```python
from build123d import *

# Parameters (mm, degrees)
SKETCH2_R           = 2.5
BOSS_EXTRUDE1_DEPTH = 2.5
CIRPATTERN1_COUNT   = 3


with BuildPart() as part:
    # Sketch1 → Revolve1 (revolve)
    with BuildSketch(Plane.XY, mode=Mode.PRIVATE) as revolve1_sk:
        Polygon((49.97067965, 0), (52.495498156, 10), (44.195498156, 10), (40, 5), (0, 5), (0, 0), align=None)
    revolve(revolve1_sk.sketch.rotate(Axis((-81.869594145, 0, 0), (1, 0, 0)), 90), axis=Axis((-81.869594145, 0, 0), (1, 0, 0)))



with BuildPart() as body_2:
    # Sketch2 → Revolve2 (revolve)
    with BuildSketch(Plane.XY, mode=Mode.PRIVATE) as revolve2_sk:
        with Locations((55, 31.25)):
            Circle(SKETCH2_R)
    revolve(revolve2_sk.sketch.rotate(Axis((0, 0, 0), (1, 0, 0)), 270), axis=Axis((0, 0, 0), (1, 0, 0)))


with BuildPart() as part_1:
    add(part.part)

    add(body_2.part)  # Boss-Extrude1 merges body 2
    # Sketch3 → Boss-Extrude1 (add, symmetric)
    with BuildSketch(Plane.XY):
        Polygon((51.6, 9.2), (49.554391748, 9.2), (53.974391748, 29.779681075), (56.02, 29.779681075), align=None)
    boss_extrude1 = extrude(amount=BOSS_EXTRUDE1_DEPTH, both=True)

    # CirPattern1: Boss-Extrude1 ×3 about axis
    cirpattern1_axis = Axis((0, 0, 0), (1, 0, 0))
    for i in range(1, CIRPATTERN1_COUNT):
        add(boss_extrude1.rotate(cirpattern1_axis, i * 360 / CIRPATTERN1_COUNT))


solid = part_1.part
```
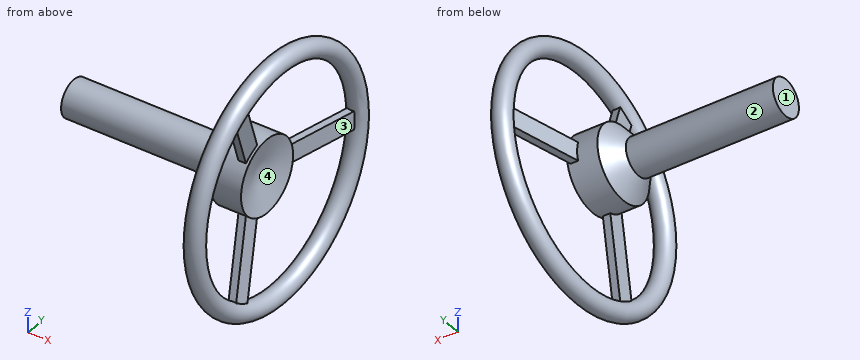
Geometry: final body of the model. Coordinates: model frame, mm. Face numbers are marked on the shaded views. Round coordinates to 2 decimals unless told otherwise and drop trailing zeros. Order: outer loops, then holes, each group sorted by start corner. A loop starts at its lowest first (then second) coordinate and runs counter-clockwise, first axis right, second up. Notation, with made-up numbers: (-37, 44) -> (-10, 44) arc R13 ccw to (-10, 57) -> close; hole circle Ø6 at (42.5, 88). An arc over 180 degrees is marked (long way). Write each question's results on one line, items separated by ' | '.
Q1. Ray query, line 1 along X through (y, z) = (-13.5, 22); line 2 along X through (y, z) = (7, -7); line 3 along Y through (x, z) = (48.5, 3). Return the intervals inside material, ascending.
Response values:
line 1: 53.12 to 55.17 | line 2: 44.11 to 52.47 | line 3: -9.54 to 9.54
Q2. Section query A-A (x = 25.5). Output: boundary loops of the cut face in (y, z).
Response values:
outline: circle Ø10 at (0, 0)
Q3. Pin query (flat end, axial travel): pin 1 Ø3 at (y, z) = (-15.5, 23) entering from +X; pin 2 Ø12 at (y, z) = (-26, 7) entering from +X; pin 3 Ø1.8 at (x, y) = (53, 19.5) entering from +Z; pin 4 Ø7 at (x, y) = (52.5, 21.5) entering from -Z. Return the tip coordinate at first contact, or that it passes through.
Response values:
pin 1: x = 56.48 | pin 2: x = 57.5 | pin 3: z = 27.5 | pin 4: z = -28.11
Q4. Pull-direction query (Y, two-part tool) for the marked faces 1, 2, 3 and 4; classes: released by +Y, released by -Y, zero draft, split by the parting line, or undercut.
Response values:
face 1: zero draft | face 2: split by the parting line | face 3: undercut | face 4: undercut
Q5. Section query D-D (x = 46.5). Output: boundary loops of the cut face in (y, z).
Response values:
outline: circle Ø20 at (0, 0)
Q6. Section query B-B (z = 6). Count the separate pieces of the cut face and the enclosed holes in it, and give its area (3 significant figures).
Response values:
separate pieces: 3 | enclosed holes: 0 | area: 197 mm²
